Job drawing, mm, ordinate dimensions from the low corner. One solid piece. A direction names the side the tool comes from. Round coordinates to 2 decimals unless told otherwise and drop trailing zeros. Write each loop counter-clockwise with the first axis right and the second up, starting at its lowest first coordinate (ties: lowest second). Pieces come first, ordered by that corner, then holes.
1) Drill centre lines: L1, parallel to X at y = 109.5, z = 22.5 (1 decimal); L2, parallel to Z at x = 154, y = 116; L3, parallel to X at y = 76.5, z = 22.25 (1 decimal). Where is each one in solid material? Low to high.
2) Pull direction X, two halves, no side cores. Call the marked faces 1, 2 and 3: +X half, -X half, draft (parallel to the pull), parting line (faces both ways), or undercut.
3) Saw through at D-D on y = 55.5. Write the cut outline in (x, z).
4) Saw through at A-A on x = 96.5. Write the cut outline in (y, z), and give its area (3 significant figures).
5) Saw through at B-B on z = 23. Write the cut outline in (x, y) (1 decimal), and give its area (3 significant figures).
6) Saw through at C-C on x = 154. Write the cut outline in (y, z).
7) Flat gauge pins, fed straight in: pin 1 (1.5 mm diameter, centred on x = 36, z = 16, fed in from -Y); pin 2 (5 mm diameter, centred on y = 33, z = 13.5, fed in from +X) (1 decimal); pin 3 (9 mm diameter, centred on x = 86.5, z = 15, fed in from -Y); pin 4 (12 mm diameter, centred on y = 44.5, z = 11, fed in from -X). Where does each tip first touch, or does it go through?
8) Which spindle directions (+Z, -Z, +X, -X, +Y, -Y) get a long thin tool onto all of the face, cutting with end or side? Do the marked faces 4 and 5. Say none if no direction does.
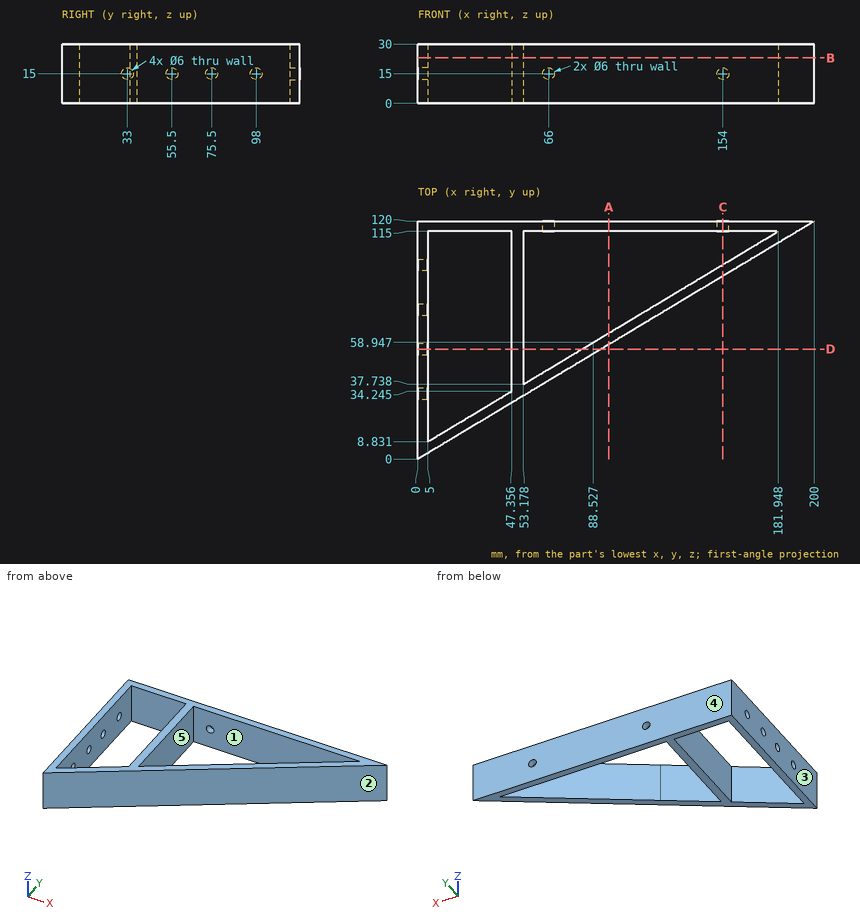
Completed:
1. L1: x = 0 to 5, 47.4 to 53.2, 172.8 to 182.5
1. L2: z = 0 to 12, 18 to 30
1. L3: x = 0 to 5, 47.4 to 53.2, 117.8 to 127.5
2. face 1: undercut
2. face 2: +X half
2. face 3: -X half
3. outline: (0, 0) - (5, 0) - (5, 12) - (0, 12) - close; (0, 18) - (5, 18) - (5, 30) - (0, 30) - close; (47.36, 0) - (53.18, 0) - (53.18, 30) - (47.36, 30) - close; (82.78, 0) - (92.5, 0) - (92.5, 30) - (82.78, 30) - close
4. outline: (57.9, 0) - (63.73, 0) - (63.73, 30) - (57.9, 30) - close; (115, 0) - (120, 0) - (120, 30) - (115, 30) - close
4. area: 325 mm2
5. outline: (0, 0) - (200, 120) - (0, 120) - close; hole (5, 8.8) - (47.4, 34.2) - (47.4, 115) - (5, 115) - close; hole (53.2, 37.7) - (181.9, 115) - (53.2, 115) - close
5. area: 3,070 mm2
6. outline: (92.4, 0) - (98.23, 0) - (98.23, 30) - (92.4, 30) - close; (115, 0) - (120, 0) - (120, 12) - (115, 12) - close; (115, 18) - (120, 18) - (120, 30) - (115, 30) - close
7. pin 1: stops at y = 21.15
7. pin 2: stops at x = 59.2
7. pin 3: stops at y = 49.2
7. pin 4: stops at x = 0
8. face 4: +Z, -Z, +X, -X, +Y
8. face 5: +Z, -Z
